```python
from build123d import *

# Parameters (mm, degrees)
SKETCH1_W           = 100
SKETCH1_H           = 50
BOSS_EXTRUDE1_DEPTH = 5
SKETCH2_W           = 130
SKETCH2_H           = 15
BOSS_EXTRUDE2_DEPTH = 10
SKETCH3_W           = 130
SKETCH3_H           = 15
BOSS_EXTRUDE3_DEPTH = 10
SKETCH4_R           = 2
CUT_EXTRUDE1_DEPTH  = 97.695398029
SKETCH5_R           = 2
CUT_EXTRUDE2_DEPTH  = 97.695398029
SKETCH7_W           = 120
SKETCH7_H           = 5
BOSS_EXTRUDE4_DEPTH = 15
SKETCH8_W           = 5
SKETCH8_H           = 15
BOSS_EXTRUDE5_DEPTH = 10
SKETCH11_W          = 120
SKETCH11_H          = 5
BOSS_EXTRUDE6_DEPTH = 15
SKETCH12_W          = 5
SKETCH12_H          = 15
BOSS_EXTRUDE7_DEPTH = 10


with BuildPart() as part:
    # Sketch1 → Boss-Extrude1 (new body)
    with BuildSketch(Plane(origin=(0, 0, 0), x_dir=(1, 0, 0), z_dir=(0, 1, 0))):
        Rectangle(SKETCH1_W, SKETCH1_H)
    extrude(amount=BOSS_EXTRUDE1_DEPTH)

    # Sketch2 → Boss-Extrude2 (add)
    with BuildSketch(Plane.XY.offset(25)):
        with Locations((0, 7.5)):
            Rectangle(SKETCH2_W, SKETCH2_H)
    extrude(amount=BOSS_EXTRUDE2_DEPTH)

    # Sketch3 → Boss-Extrude3 (add)
    with BuildSketch(Plane(origin=(0, 0, -25), x_dir=(-1, 0, 0), z_dir=(0, 0, -1))):
        with Locations((0, 7.5)):
            Rectangle(SKETCH3_W, SKETCH3_H)
    extrude(amount=BOSS_EXTRUDE3_DEPTH)

    # Sketch4 → Cut-Extrude1 (cut, through all)
    with BuildSketch(Plane.XY.offset(35)):
        with Locations((-60, 4)):
            Circle(SKETCH4_R)
    extrude(amount=-CUT_EXTRUDE1_DEPTH, mode=Mode.SUBTRACT)

    # Sketch5 → Cut-Extrude2 (cut, through all)
    with BuildSketch(Plane.XY.offset(35)):
        with Locations((60, 4)):
            Circle(SKETCH5_R)
    extrude(amount=-CUT_EXTRUDE2_DEPTH, mode=Mode.SUBTRACT)

    # Sketch7 → Boss-Extrude4 (add)
    with BuildSketch(Plane.XY.offset(35)):
        with Locations((0, 2.5)):
            Rectangle(SKETCH7_W, SKETCH7_H)
    extrude(amount=BOSS_EXTRUDE4_DEPTH)

    # Sketch8 → Boss-Extrude5 (add)
    with BuildSketch(Plane(origin=(0, 5, 0), x_dir=(1, 0, 0), z_dir=(0, 1, 0))):
        with Locations((-57.5, -42.5)):
            Rectangle(SKETCH8_W, SKETCH8_H)
        with Locations((57.5, -42.5)):
            Rectangle(SKETCH8_W, SKETCH8_H)
    extrude(amount=BOSS_EXTRUDE5_DEPTH)

    # Sketch11 → Boss-Extrude6 (add)
    with BuildSketch(Plane(origin=(0, 0, -35), x_dir=(-1, 0, 0), z_dir=(0, 0, -1))):
        with Locations((0, 2.5)):
            Rectangle(SKETCH11_W, SKETCH11_H)
    extrude(amount=BOSS_EXTRUDE6_DEPTH)

    # Sketch12 → Boss-Extrude7 (add)
    with BuildSketch(Plane(origin=(0, 5, 0), x_dir=(1, 0, 0), z_dir=(0, 1, 0))):
        with Locations((-57.5, 42.5)):
            Rectangle(SKETCH12_W, SKETCH12_H)
        with Locations((57.5, 42.5)):
            Rectangle(SKETCH12_W, SKETCH12_H)
    extrude(amount=BOSS_EXTRUDE7_DEPTH)


solid = part.part
```
Could you check a few things on this model? Use its own coordinates, in mm. A direction names the side the tool comes from. Round coordinates to 2 decimals unless told otherwise and drop trailing zeros. Loops run counter-clockwise (first coordinate to the right, second up) from the corner with the lowest first, then second, coordinate; pieces in that order, holes last. Notation, with made-up numbers: (40, 36) - (48, 36) arc R19 cw to (48, 49) - close; hole circle Ø6 at (-9, -2.5). An arc over 180 degrees is marked (long way). Use CSV: the item, a comma, the result in double quotes.
Item 1: For faces 1 (the cylindrical face through (61.847, 3.234, 30.07)), 2 (the flat face through (-60, 7, -42)), 3 (the flat face through (1, 5, -42)), 4 (the flat face through (62, 8, 35)), 5 (the flat face through (-1, 10, 35)), which set-ups out of +Z, -Z, +X, -X, +Y, -Y let a thin tool reach every point of the face, with its end or its side?
Here are the results:
face 1,"none"
face 2,"-Z, -X, +Y, -Y"
face 3,"-Z, +Y"
face 4,"+Z, +X, +Y, -Y"
face 5,"+Z, +Y"
Item 2: If we section it at B-B on y = 11: List the corners of the cut face in (x, z) for me.
Here are the results:
outline,"(-65, -35) - (-60, -35) - (-60, -50) - (-55, -50) - (-55, -35) - (55, -35) - (55, -50) - (60, -50) - (60, -35) - (65, -35) - (65, -25) - (-65, -25) - close; (-65, 25) - (65, 25) - (65, 35) - (60, 35) - (60, 50) - (55, 50) - (55, 35) - (-55, 35) - (-55, 50) - (-60, 50) - (-60, 35) - (-65, 35) - close"
Item 3: If we section it at A-A on x = 53: List the corners of the cut face in (y, z) for me, then the cut area to 3 significant figures.
Here are the results:
outline,"(0, -50) - (5, -50) - (5, -35) - (15, -35) - (15, -25) - (0, -25) - close; (0, 25) - (15, 25) - (15, 35) - (5, 35) - (5, 50) - (0, 50) - close"
area,"450 mm²"
Item 4: If we section it at C-C on z = -43: List the corners of the cut face in (x, y) for me, then the cut area to 3 significant figures.
Here are the results:
outline,"(-60, 0) - (60, 0) - (60, 15) - (55, 15) - (55, 5) - (-55, 5) - (-55, 15) - (-60, 15) - close"
area,"700 mm²"
Item 5: Will these pins go through, and if not, where does the flat tip stop? pin 1 (2 mm diameter, centred on x = -6, y = 12, fed in from -Z); pin 2 (5.5 mm diameter, centred on y = 2, z = -10.5, fed in from +X); pin 3 (8 mm diameter, centred on y = 9, z = 45.5, fed in from +X).
Here are the results:
pin 1,"stops at z = -35"
pin 2,"stops at x = 50"
pin 3,"stops at x = 60"
Item 6: If we section it at D-D on x = -42.5: List the corners of the cut face in (y, z) for me, then the cut area to 3 significant figures.
Here are the results:
outline,"(0, -50) - (5, -50) - (5, -35) - (15, -35) - (15, -25) - (5, -25) - (5, 25) - (15, 25) - (15, 35) - (5, 35) - (5, 50) - (0, 50) - close"
area,"700 mm²"
Item 7: I need wall thicknesses on L1, parallel to X at y = 4, z = 28.5; L2, parallel to Z at x = 42, y = 11; L3, parallel to Y at x = 60, z = -32.25. Which ranges of each line are inside material? Lowest first, please. Write a range as [from, to].
Here are the results:
L1,"x = [-65, -62], [-58, 58], [62, 65]"
L2,"z = [-35, -25], [25, 35]"
L3,"y = [0, 2], [6, 15]"
Item 8: If we mould it in two halves opening along Z, with no side actions, what happens to faces 6 (the cylindrical face through (-58.153, 3.234, -29.93)), 7 (the flat face through (55, 10, -42)), 8 (the flat face through (63, 8, -35))? For each: pulls with the +Z half, pulls with the -Z half, needs draft (parallel to the pull), parting line crosses it, or undercut.
Here are the results:
face 6,"undercut"
face 7,"needs draft"
face 8,"pulls with the -Z half"
